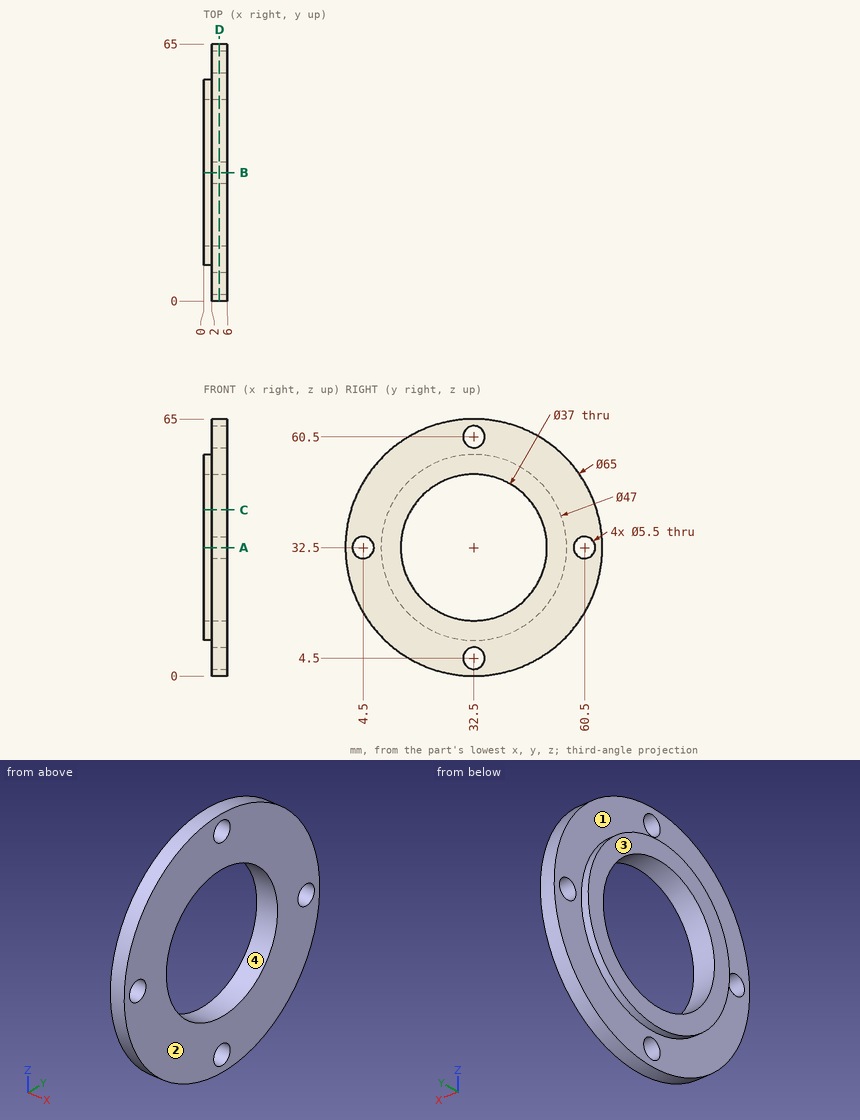
Input: dimensioned drawing with shaded views. Units: mm. Origin: part minimum x, y, z. A direction names the side the tool comes from. Round coordinates to 2 decimals unless told otherwise and drop trailing zeros. Order: outer loops, then holes, each group sorted by start corner. A loop starts at its lowest first (then second) coordinate and runs counter-clockwise, first axis right, second up. Notation, with made-up numbers: (9, -16.5) - (50, -16.5) arc R26 cw to (50, 6.5) - close; hole circle Ø1 at (73, -3). An arc over 180 degrees is marked (long way). Write item = value, one per line. Start each with the question number.
Q1. Pin query (flat end, axial travel): pin 1 (6 mm diameter, centred on y = 16.5, z = 8.5, fed in from -X); pin 2 (1.5 mm diameter, centred on x = 5, z = 11, fed in from +Y); pin 3 (1.5 mm diameter, centred on x = 2.5, z = 38, fed in from +Y). Return the tip coordinate at first contact, or that it passes through.
Q2. Pull-direction query (Y, two-part tool) for the marked faces 3 and 4; classes: +Y half, -Y half, draft (parallel to the pull), parting line (faces both ways), or undercut.
Q3. Cut plane A-A on z = 32.5. Return the cut outline in (x, y).
Q4. Ray query, line 1 (Z direction, x = 2.4, y = 32.5); line 2 (Z direction, x = 4.15, y = 26); line 3 (Y direction, x = 5, z = 47). Return the intervals inside material, ascending. Write a range as from..to.
Q5. Cut plane D-D on x = 4. Return the cut outline in (y, z), and give its area (3 significant figures).
Q6. Access query for the marked faces 1 and 2. Directions: +Z, -Z, +X, -X, +Y, -Y. A direction counts if a zero-diameter tool reaches every point of the face in a straight line with its end or side. Return the directions, or none.
Q7. Cut plane C-C on z = 42. Return the cut outline in (x, y).
Outcome:
q1.pin_1 = 2
q1.pin_2 = 57.51
q1.pin_3 = 64.65
q2.face_3 = draft
q2.face_4 = undercut
q3.outline = (0, 9) - (2, 9) - (2, 7.25) - (6, 7.25) - (6, 14) - (0, 14) - close; (0, 51) - (6, 51) - (6, 57.75) - (2, 57.75) - (2, 56) - (0, 56) - close; (2, 0) - (6, 0) - (6, 1.75) - (2, 1.75) - close; (2, 63.25) - (6, 63.25) - (6, 65) - (2, 65) - close
q4.line_1 = 0..1.75, 7.25..14, 51..57.75, 63.25..65
q4.line_2 = 0.66..15.18, 49.82..64.34
q4.line_3 = 3.41..21.01, 43.99..61.59
q5.outline = circle Ø65 at (32.5, 32.5); hole circle Ø5.5 at (4.5, 32.5); hole circle Ø37 at (32.5, 32.5); hole circle Ø5.5 at (32.5, 4.5); hole circle Ø5.5 at (32.5, 60.5); hole circle Ø5.5 at (60.5, 32.5)
q5.area = 2,150 mm^2
q6.face_1 = -X
q6.face_2 = +Z, -Z, +X, +Y, -Y
q7.outline = (0, 11.01) - (2, 11.01) - (2, 1.42) - (6, 1.42) - (6, 16.63) - (0, 16.63) - close; (0, 48.37) - (6, 48.37) - (6, 63.58) - (2, 63.58) - (2, 53.99) - (0, 53.99) - close
